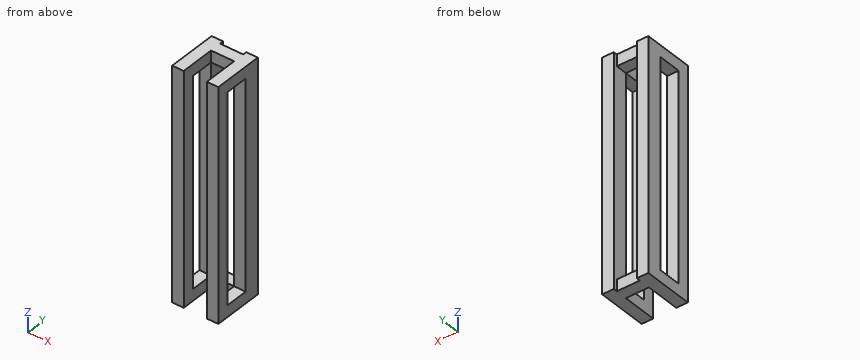
from build123d import *

# Parameters (mm, degrees)
F0_W     = 3.81
F0_H     = 3.81
F0_W_2   = 7.62
F0_H_2   = 68.58
F1_DEPTH = 3.81
F2_DEPTH = 1.27
F3_DEPTH = 15.24
F4_W     = 3.81
F4_H     = 3.81
F5_DEPTH = 68.58
F6_W     = 3.81
F6_H     = 3.81
F7_DEPTH = 68.58


with BuildPart() as f1:
    # F0 (on Front) → F1 (new body)
    with BuildSketch(Plane.XZ):
        with Locations((-51.6441376173, 83.97309774)):
            Rectangle(F0_W, F0_H)
        with Locations((-45.9291376173, 83.97309774)):
            Rectangle(F0_W_2, F0_H)
        with Locations((-40.2141376173, 83.97309774)):
            Rectangle(F0_W, F0_H)
        with Locations((-40.2141376173, 47.77809774)):
            Rectangle(F0_W, F0_H_2)
        with Locations((-51.6441376173, 47.77809774)):
            Rectangle(F0_W, F0_H_2)
        with Locations((-51.6441376173, 11.58309774)):
            Rectangle(F0_W, F0_H)
        with Locations((-45.9291376173, 11.58309774)):
            Rectangle(F0_W_2, F0_H)
        with Locations((-40.2141376173, 11.58309774)):
            Rectangle(F0_W, F0_H)
    extrude(amount=F1_DEPTH)

    # F0 (on Front) → F2 (join)
    with BuildSketch(Plane.XZ):
        with Locations((-51.6441376173, 47.77809774)):
            Rectangle(F0_W, F0_H_2)
        with Locations((-51.6441376173, 83.97309774)):
            Rectangle(F0_W, F0_H)
        with Locations((-40.2141376173, 83.97309774)):
            Rectangle(F0_W, F0_H)
        with Locations((-40.2141376173, 47.77809774)):
            Rectangle(F0_W, F0_H_2)
        with Locations((-40.2141376173, 11.58309774)):
            Rectangle(F0_W, F0_H)
        with Locations((-51.6441376173, 11.58309774)):
            Rectangle(F0_W, F0_H)
    extrude(amount=-F2_DEPTH)

    # F0 (on Front) → F3 (join)
    with BuildSketch(Plane.XZ):
        with Locations((-51.6441376173, 83.97309774)):
            Rectangle(F0_W, F0_H)
        with Locations((-40.2141376173, 83.97309774)):
            Rectangle(F0_W, F0_H)
        with Locations((-51.6441376173, 11.58309774)):
            Rectangle(F0_W, F0_H)
        with Locations((-40.2141376173, 11.58309774)):
            Rectangle(F0_W, F0_H)
    extrude(amount=F3_DEPTH)

    # F4 (on face) → F5 (join)
    with BuildSketch(Plane(origin=(0, 0, 82.06809774), x_dir=(1, 0, 0), z_dir=(0, 0, -1))):
        with Locations((-51.6441376173, 13.335)):
            Rectangle(F4_W, F4_H)
    extrude(amount=F5_DEPTH)

    # F6 (on face) → F7 (join)
    with BuildSketch(Plane(origin=(0, 0, 82.06809774), x_dir=(1, 0, 0), z_dir=(0, 0, -1))):
        with Locations((-40.2141376173, 13.335)):
            Rectangle(F6_W, F6_H)
    extrude(amount=F7_DEPTH)


solid = f1.part
Work out the finished part from the listing and answer in its coordinate system (mm). Give positions to 0.01 mm unless a question says otherwise; leave off trailing zeros. Loops run counter-clockwise (first coordinate to the right, second up) from the corner with the lowest first, then second, coordinate; pieces in that order, holes last. Notation, with made-up numbers: (85.5, -24.5) - (113.5, -24.5) arc R38 cw to (113.5, 14.5) - close; hole circle Ø11 at (-38, -22.5). An arc over 180 degrees is marked (long way). Answer in a Markdown table with one row per item.
(1) Consider L1, parallel to Z at x = -40.25, y = -5; L2, parallel to X at y = -14.5, z = 28.5; L3, parallel to Y at x = -42, z = 23. Determine where each line is inside the solid, lowest interval first. Write a range as [from, to].
Results list:
| item | result |
|---|---|
| L1 | z = [9.68, 13.49], [82.07, 85.88] |
| L2 | x = [-53.55, -49.74], [-42.12, -38.31] |
| L3 | y = [-15.24, -11.43], [-3.81, 1.27] |
(2) Section D-D (x = -50.5) is taken. Give the vertices of the cut face in (y, z), and give its area (3 significant figures).
Results list:
| item | result |
|---|---|
| outline | (-15.24, 9.68) - (1.27, 9.68) - (1.27, 85.88) - (-15.24, 85.88) - close; hole (-11.43, 13.49) - (-3.81, 13.49) - (-3.81, 82.07) - (-11.43, 82.07) - close |
| area | 735 mm² |
(3) Flat-ended cylindrical pins translate along their axes: pin 1 Ø9 at (y, z) = (-8.5, 32.5) entering from +X; pin 2 Ø1.9 at (x, z) = (-46.5, 12) entering from +Y; pin 3 Ø4 at (x, z) = (-46.5, 83.5) entering from -Y. Find the tip coordinate at first contact, or state that the pin passes through.
Results list:
| item | result |
|---|---|
| pin 1 | stops at x = -38.31 |
| pin 2 | stops at y = 0 |
| pin 3 | stops at y = -3.81 |
(4) Section C-C (x = -46.25) is taken. Give the vertices of the cut face in (y, z).
Results list:
| item | result |
|---|---|
| outline | (-3.81, 9.68) - (0, 9.68) - (0, 13.49) - (-3.81, 13.49) - close; (-3.81, 82.07) - (0, 82.07) - (0, 85.88) - (-3.81, 85.88) - close |
(5) Section A-A (z = 52) is taken. Give the vertices of the cut face in (x, y), and give its area (3 significant figures).
Results list:
| item | result |
|---|---|
| outline | (-53.55, -15.24) - (-49.74, -15.24) - (-49.74, -11.43) - (-53.55, -11.43) - close; (-53.55, -3.81) - (-49.74, -3.81) - (-49.74, 1.27) - (-53.55, 1.27) - close; (-42.12, -15.24) - (-38.31, -15.24) - (-38.31, -11.43) - (-42.12, -11.43) - close; (-42.12, -3.81) - (-38.31, -3.81) - (-38.31, 1.27) - (-42.12, 1.27) - close |
| area | 67.7 mm² |
(6) Section B-B (y = -13) is taken. Give the vertices of the cut face in (x, z).
Results list:
| item | result |
|---|---|
| outline | (-53.55, 9.68) - (-49.74, 9.68) - (-49.74, 85.88) - (-53.55, 85.88) - close; (-42.12, 9.68) - (-38.31, 9.68) - (-38.31, 85.88) - (-42.12, 85.88) - close |
